Could you check a few things on this model? Use its own coordinates, in mm. A direction names the side the tool comes from. Coordinates: 2 decimals unless noted, no trailing zeros. Order: outer loops, then holes, each group sorted by start corner. A loop starts at its lowest first (then second) coordinate and runs counter-clockwise, first axis right, second up. Notation, with made-up numbers: (-40, 38.25) -> (-3, 38.25) arc R19 ccw to (-3, 65.25) -> close; hole circle Ø1 at (65.5, 19.25). An arc over 180 degrees is marked (long way). Use a Markdown table: item, result. Add a question column.
1) If we section it at D-D (z = -48): Write out the boundary of the cut face in (x, y), plus the area to 3 significant figures.
2) Which directions (+Z, -Z, +X, -X, +Y, -Y) give clear straight access to the entire face, cutting with the end or side of a thin tool? Please do faces 1 (the flat face through (1, 77, -41.275)), 2 (the flat face through (1, 77, 34.925)), 3 (the flat face through (-41, 11, -130.175)), 4 (the flat face through (-1, 0, -38)), 5 (the flat face through (-41, -75, -28.575)).
3) Will these pins go through, and if not, where does the flat tip stop? pin 1 Ø1.9 at (x, z) = (6.5, -38.5) entering from -Y; pin 2 Ø1 at (x, y) = (30, 68) entering from +Z (3 decimals); pin 3 Ø23 at (x, y) = (-15.5, 83) entering from -Z (3 decimals).
4) If I drill on L1, parallel to Z at x = -41, y = -127 (3 decimals); L2, parallel to X at y = -94, z = -94; L3, parallel to X at y = 101, z = 39, over which ranges is the centre line in solid material (lowest first)? Write a range as [from, to].
5) If we section it at A-A (x = 0): Write out the boundary of the cut face in (y, z) (3 decimals).
6) If we section it at C-C (x = 30.5): Write out the boundary of the cut face in (y, z) (3 decimals).
7) If we section it at B-B (y = -88.9): Give the number of separate pieces and of enclosed holes in the cut face, plus the area to 3 significant figures.
8) Thinking about a two-plate mould opening in X: for faces 6 (the flat face through (1, 77, -34.925)), 7 (the flat face through (44.45, 32, 2)), 8 (the flat face through (41, 0, 0)), which applies, +X half, -X half, draft (parallel to the pull), parting line (faces both ways), or undercut?
```python
from build123d import *

# Parameters (mm, degrees)
F0_R     = 7.9375
F0_R_2   = 6.35
F1_DEPTH = 44.45
F2_W     = 76.2
F2_H     = 88.9
F2_H_2   = 69.85
F3_DEPTH = 304.801
F4_W     = 76.2
F4_H     = 148.997045
F4_R     = 19.05
F5_DEPTH = 171.451


with BuildPart() as f1:
    # F0 (on Right) → F1 (new body, symmetric)
    with BuildSketch(Plane.YZ):
        with BuildLine():
            Line((152.4, 130.175), (-127, 130.175))
            ThreePointArc((-127, 130.175), (-144.960512, 122.735512), (-152.4, 104.775))
            Line((-152.4, 104.775), (-152.4, 53.975))
            ThreePointArc((-152.4, 53.975), (-144.960512, 36.014488), (-127, 28.575))
            Line((-127, 28.575), (-25.4, 28.575))
            ThreePointArc((-25.4, 28.575), (-7.439488, 21.135512), (0, 3.175))
            Line((0, 3.175), (0, -3.175))
            ThreePointArc((0, -3.175), (-7.439488, -21.135512), (-25.4, -28.575))
            Line((-25.4, -28.575), (-127, -28.575))
            ThreePointArc((-127, -28.575), (-144.960512, -36.014488), (-152.4, -53.975))
            Line((-152.4, -53.975), (-152.4, -104.775))
            ThreePointArc((-152.4, -104.775), (-144.960512, -122.735512), (-127, -130.175))
            Line((-127, -130.175), (152.4, -130.175))
            Line((152.4, -130.175), (152.4, 130.175))
        make_face()
        with Locations((-88.9, -79.375)):
            Circle(F0_R, mode=Mode.SUBTRACT)
        with Locations((-127, 79.375)):
            Circle(F0_R_2, mode=Mode.SUBTRACT)
    extrude(amount=F1_DEPTH, both=True)

    # F2 (on face) → F3 (cut, through all)
    with BuildSketch(Plane(origin=(0, 152.4, 0), x_dir=(-1, 0, 0), z_dir=(0, 1, 0))):
        with Locations((0, 85.725)):
            Rectangle(F2_W, F2_H)
        Rectangle(F2_W, F2_H_2)
        with Locations((0, -85.725)):
            Rectangle(F2_W, F2_H)
    extrude(amount=-F3_DEPTH, mode=Mode.SUBTRACT)

    # F4 (on face) → F5 (cut, through all)
    with BuildSketch(Plane.XY.offset(41.275)):
        with Locations((0, -74.498522)):
            Rectangle(F4_W, F4_H)
        with Locations((0, 101.6)):
            Circle(F4_R)
    extrude(amount=-F5_DEPTH, mode=Mode.SUBTRACT)


solid = f1.part
```
Answer sheet:
| question | item | result |
|---|---|---|
| 1 | outline | (-44.45, -151.69) -> (-38.1, -151.69) -> (-38.1, 152.4) -> (-44.45, 152.4) -> close; (38.1, -151.69) -> (44.45, -151.69) -> (44.45, 152.4) -> (38.1, 152.4) -> close |
| 1 | area | 3,860 mm2 |
| 2 | face 1 | -Z, +Y, -Y |
| 2 | face 2 | +Y, -Y |
| 2 | face 3 | -Z, +X, -X, +Y, -Y |
| 2 | face 4 | +Z, -Z, -Y |
| 2 | face 5 | +X, -X, -Y |
| 3 | pin 1 | y = 0 |
| 3 | pin 2 | z = 41.275 |
| 3 | pin 3 | z = -41.275 |
| 4 | L1 | [-130.175, -28.575], [28.575, 73.025], [85.725, 130.175] |
| 4 | L2 | [-44.45, -38.1], [38.1, 44.45] |
| 4 | L3 | [-44.45, -19.04], [19.04, 44.45] |
| 5 | outline | (0, -41.275) -> (82.55, -41.275) -> (82.55, -34.925) -> (0, -34.925) -> close; (0, 34.925) -> (82.55, 34.925) -> (82.55, 41.275) -> (0, 41.275) -> close; (120.65, -41.275) -> (152.4, -41.275) -> (152.4, -34.925) -> (120.65, -34.925) -> close; (120.65, 34.925) -> (152.4, 34.925) -> (152.4, 41.275) -> (120.65, 41.275) -> close |
| 6 | outline | (0, -41.275) -> (152.4, -41.275) -> (152.4, -34.925) -> (0, -34.925) -> close; (0, 34.925) -> (152.4, 34.925) -> (152.4, 41.275) -> (0, 41.275) -> close |
| 7 | separate pieces | 6 |
| 7 | enclosed holes | 0 |
| 7 | area | 2,380 mm2 |
| 8 | face 6 | undercut |
| 8 | face 7 | +X half |
| 8 | face 8 | draft |
